```python
from build123d import *

# Parameters (mm, degrees)
F0_W     = 47.6
F0_H     = 47.6
F1_DEPTH = 1.6
F2_W     = 3.3
F2_H     = 47.6
F3_DEPTH = 3.3
F4_W     = 47.6
F4_H     = 3.3
F5_DEPTH = 3.3


with BuildPart() as f1:
    # F0 (on Top) → F1 (new body, symmetric)
    with BuildSketch(Plane.XY):
        Rectangle(F0_W, F0_H)
        with BuildLine():
            ThreePointArc((-8.313844, 3.7), (0, 9.1), (8.313844, 3.7))
            Line((8.313844, 3.7), (10.8, 3.7))
            ThreePointArc((10.8, 3.7), (14.5, 0), (10.8, -3.7))
            Line((10.8, -3.7), (8.313844, -3.7))
            ThreePointArc((8.313844, -3.7), (0, -9.1), (-8.313844, -3.7))
            Line((-8.313844, -3.7), (-10.8, -3.7))
            ThreePointArc((-10.8, -3.7), (-14.5, 0), (-10.8, 3.7))
            Line((-10.8, 3.7), (-8.313844, 3.7))
        make_face(mode=Mode.SUBTRACT)
    extrude(amount=F1_DEPTH, both=True)

    # F2 (on face) → F3 (join)
    with BuildSketch(Plane.XY.offset(1.6)):
        with Locations((-22.15, 0)):
            Rectangle(F2_W, F2_H)
        with Locations((22.15, 0)):
            Rectangle(F2_W, F2_H)
    extrude(amount=F3_DEPTH)

    # F4 (on face) → F5 (join)
    with BuildSketch(Plane(origin=(0, 0, -1.6), x_dir=(1, 0, 0), z_dir=(0, 0, -1))):
        with Locations((0, -22.15)):
            Rectangle(F4_W, F4_H)
        with Locations((0, 22.15)):
            Rectangle(F4_W, F4_H)
    extrude(amount=F5_DEPTH)


solid = f1.part
```
Here's how the part is built. I have some questions about the finished solid (model axes, mm). A direction names the side the tool comes from. Give positions to 0.01 mm unless a question says otherwise; leave off trailing zeros. Order: outer loops, then holes, each group sorted by start corner. A loop starts at its lowest first (then second) coordinate and runs counter-clockwise, first axis right, second up. Notation, with made-up numbers: (35.25, 72.25) -> (83.25, 72.25) arc R28 ccw to (83.25, 97.25) -> close; hole circle Ø9 at (39, 53). An arc over 180 degrees is marked (long way). Use CSV: the item, a comma, the result in double quotes. Start each with the question number.
Item 1: If I drill on probe 1 along Y at (x, z) = (19.5, -2.75); probe 2 along Y at (x, z) = (8.5, 1.25), over which ranges is the centre line in solid material (lowest first)? Write a range as [from, to].
Item 2: Suppose I cut it at C-C (x = 6.5). List the corners of the cut face in (y, z) for me, and give its area (3 significant figures).
Item 3: Suppose I cut it at A-A (z = -4). List the corners of the cut face in (x, y) for me, and give its area (3 significant figures).
Item 4: On a 3-axis mill with a long thin cutter (end or side, diameter ignored), from which of +Z, -Z, +X, -X, +Y, -Y can I reach the whole of each face in a straight line? I mean faces 1 (the flat face through (23.8, 0, 1)), 2 (the cylindrical face through (-0.1, 9.1, 0)), 3 (the flat face through (-9, -5, 1.6)), 4 (the flat face through (0, -20.5, -3)), 5 (the flat face through (0, 22, -4.9)). Say none if no direction works.
Item 5: I'm going to push flat-ended pins straight in: P1, Ø20.5, axis at x = -1.5, y = -11, coming from the +Z side; P2, Ø3, axis at x = -5.5, y = 16, coming from the -Z side. Where does each tip first touch, or does it pass through?
Item 6: Suppose I cut it at D-D (z = 0.5). List the corners of the cut face in (x, y) for me.
Item 7: Suppose I cut it at B-B (y = 0). List the corners of the cut face in (x, z) for me, and give its area (3 significant figures).
Item 8: Thinking about a two-plate mould opening in Y: for faces 6 (the flat face through (0, -23.8, -1)), 7 (the flat face through (-23.8, 0, 1)), 8 (the flat face through (0, 20.5, -3)), which applies, pulls with the +Y half, pulls with the -Y half, needs draft (parallel to the pull), parting line crosses it, or undercut?
Answer block:
1,probe 1,"y = [-23.8, -20.5], [20.5, 23.8]"
1,probe 2,"y = [-23.8, -3.7], [3.7, 23.8]"
2,outline,"(-23.8, -4.9) -> (-20.5, -4.9) -> (-20.5, -1.6) -> (-6.37, -1.6) -> (-6.37, 1.6) -> (-23.8, 1.6) -> close; (6.37, -1.6) -> (20.5, -1.6) -> (20.5, -4.9) -> (23.8, -4.9) -> (23.8, 1.6) -> (6.37, 1.6) -> close"
2,area,"133 mm^2"
3,outline,"(-23.8, -23.8) -> (23.8, -23.8) -> (23.8, -20.5) -> (-23.8, -20.5) -> close; (-23.8, 20.5) -> (23.8, 20.5) -> (23.8, 23.8) -> (-23.8, 23.8) -> close"
3,area,"314 mm^2"
4,face 1,"+Z, -Z, +X, +Y, -Y"
4,face 2,"+Z, -Z"
4,face 3,"+Z, +Y, -Y"
4,face 4,"-Z, +X, -X"
4,face 5,"-Z, +X, -X, +Y, -Y"
5,P1,"stops at z = 1.6"
5,P2,"stops at z = -1.6"
6,outline,"(-23.8, -23.8) -> (23.8, -23.8) -> (23.8, 23.8) -> (-23.8, 23.8) -> close; hole (-10.8, -3.7) -> (-8.31, -3.7) arc R9.1 ccw to (8.31, -3.7) -> (10.8, -3.7) arc R3.7 ccw to (10.8, 3.7) -> (8.31, 3.7) arc R9.1 ccw to (-8.31, 3.7) -> (-10.8, 3.7) arc R3.7 ccw to start"
7,outline,"(-23.8, -1.6) -> (-14.5, -1.6) -> (-14.5, 1.6) -> (-20.5, 1.6) -> (-20.5, 4.9) -> (-23.8, 4.9) -> close; (14.5, -1.6) -> (23.8, -1.6) -> (23.8, 4.9) -> (20.5, 4.9) -> (20.5, 1.6) -> (14.5, 1.6) -> close"
7,area,"81.3 mm^2"
8,face 6,"pulls with the -Y half"
8,face 7,"needs draft"
8,face 8,"undercut"
